Build history of the part. All positions in model axes, mm. A direction names the side the tool comes from. Give positions to 0.01 mm unless a question says otherwise; leave off trailing zeros. Loops run counter-clockwise (first coordinate to the right, second up) from the corner with the lowest first, then second, coordinate; pieces in that order, holes last. Notation, with made-up numbers: M 73,-22.75 L 100,-22.75 A14 ccw 100,-7.75 Z; hole C 30.5,-39 d4. An arc over 180 degrees is marked long. Answer as a JSON object with one key per item and string values. Group by question number.
1. Drill centre lines: line 1 along X through (y, z) = (16.5, -6.5); line 2 along Y through (x, z) = (62, -49); line 3 along Y through (x, z) = (69, -9). Where is each one in solid material? Low to high. Write a range as [from, to].
2. Mould opens along Z. For faces 4 (the face through (44, -4, -49.1)), 5 (the face through (44, -4, -20.9)), 6 (the face through (44, 7, 0)), 7 (the face through (90, 0.3, -6.4)) say: released by +Z, released by -Z, zero draft, split by the parting line, or undercut.
3. Slice it at A-A (y = 19.5). List the corners of the cut face in (x, z).
4. Drop flat-ended pins along their axis: pin 1 Ø4 at (x, z) = (78.5, -53) entering from -Y; pin 2 Ø21 at (x, z) = (59, -44) entering from +Y; pin 3 Ø2 at (x, z) = (68, -41.5) entering from -Y; pin 4 Ø14.5 at (y, z) = (16.5, -27.5) entering from +X. Give the stop position or say it passes through.
5. Slice it at B-B (z = -6). List the corners of the cut face in (x, y).
6. 3-axis set-ups, long thin cutter, end or side, ignore diameter. For faces 1 (the face through (90, 0.3, -42.2)), 2 (the face through (87, 2, -62.4)), 3 (the face through (44, -4, -72.1)): which of +Z, -Z, +X, -X, +Y, -Y reach the whole face in a straight line?
7. Slice it at C-C (y = -1). Give the number of separate pieces and of enclosed holes in the cut face, then the cut area to 3 significant figures.
from build123d import *

# Parameters (mm, degrees)
ESQUISSE1_W             = 90
ESQUISSE1_H             = 75
BOSS_EXTRU_1_DEPTH      = 3.7
ESQUISSE2_W             = 90
ESQUISSE2_H             = 2.9
ESQUISSE2_H_2           = 2
ESQUISSE2_H_3           = 0.8
BOSS_EXTRU_2_DEPTH      = 9
ENL_V_MAT_EXTRU_1_DEPTH = 118.84010353
ESQUISSE4_W             = 90
ESQUISSE4_H             = 2.9
BOSS_EXTRU_3_DEPTH      = 22
ESQUISSE5_W             = 72
ESQUISSE5_H             = 72.1
BOSS_EXTRU_4_DEPTH      = 20
CONG_1_R                = 1


with BuildPart() as part:
    # Esquisse1 → Boss.-Extru.1 (new body)
    with BuildSketch(Plane(origin=(0, 0, 0), x_dir=(1, 0, 0), z_dir=(0, 1, 0))):
        with Locations((45, 37.5)):
            Rectangle(ESQUISSE1_W, ESQUISSE1_H)
    extrude(amount=BOSS_EXTRU_1_DEPTH)

    # Esquisse2 → Boss.-Extru.2 (add)
    with BuildSketch(Plane.XZ):
        with Locations((45, -73.55)):
            Rectangle(ESQUISSE2_W, ESQUISSE2_H)
        with Locations((45, -1)):
            Rectangle(ESQUISSE2_W, ESQUISSE2_H_2)
        with Locations((45, -66.9)):
            Rectangle(ESQUISSE2_W, ESQUISSE2_H_3)
        with Locations((45, -61.1)):
            Rectangle(ESQUISSE2_W, ESQUISSE2_H_3)
        with Locations((45, -55.3)):
            Rectangle(ESQUISSE2_W, ESQUISSE2_H_3)
        with Locations((45, -49.5)):
            Rectangle(ESQUISSE2_W, ESQUISSE2_H_3)
        with Locations((45, -43.7)):
            Rectangle(ESQUISSE2_W, ESQUISSE2_H_3)
        with Locations((45, -37.9)):
            Rectangle(ESQUISSE2_W, ESQUISSE2_H_3)
        with Locations((45, -32.1)):
            Rectangle(ESQUISSE2_W, ESQUISSE2_H_3)
        with Locations((45, -26.3)):
            Rectangle(ESQUISSE2_W, ESQUISSE2_H_3)
        with Locations((45, -20.5)):
            Rectangle(ESQUISSE2_W, ESQUISSE2_H_3)
        with Locations((45, -14.7)):
            Rectangle(ESQUISSE2_W, ESQUISSE2_H_3)
        with Locations((45, -8.9)):
            Rectangle(ESQUISSE2_W, ESQUISSE2_H_3)
    extrude(amount=BOSS_EXTRU_2_DEPTH)

    # Esquisse3 → Enlèv. mat.-Extru.1 (cut, through all)
    with BuildSketch(Plane(origin=(0, 3.7, 0), x_dir=(1, 0, 0), z_dir=(0, 1, 0))):
        with BuildLine():
            Line((90, 12.6), (84.9, 12.6))
            ThreePointArc((84.9, 12.6), (82.5, 15), (84.9, 17.4))
            Line((84.9, 17.4), (90, 17.4))
            Line((90, 17.4), (90, 12.6))
        make_face()
        with BuildLine():
            Line((84.9, 57.6), (90, 57.6))
            Line((90, 57.6), (90, 62.4))
            Line((90, 62.4), (84.9, 62.4))
            ThreePointArc((84.9, 62.4), (82.5, 60), (84.9, 57.6))
        make_face()
        with BuildLine():
            Line((0, 57.6), (0, 62.4))
            Line((0, 62.4), (5.1, 62.4))
            ThreePointArc((5.1, 62.4), (7.5, 60), (5.1, 57.6))
            Line((5.1, 57.6), (0, 57.6))
        make_face()
        with BuildLine():
            Line((0, 17.4), (0, 12.6))
            Line((0, 12.6), (5.1, 12.6))
            ThreePointArc((5.1, 12.6), (7.5, 15), (5.1, 17.4))
            Line((5.1, 17.4), (0, 17.4))
        make_face()
    extrude(amount=-ENL_V_MAT_EXTRU_1_DEPTH, mode=Mode.SUBTRACT)

    # Esquisse4 → Boss.-Extru.3 (add)
    with BuildSketch(Plane(origin=(0, 3.7, 0), x_dir=(1, 0, 0), z_dir=(0, 1, 0))):
        with Locations((45, 73.55)):
            Rectangle(ESQUISSE4_W, ESQUISSE4_H)
    extrude(amount=BOSS_EXTRU_3_DEPTH)

    # Esquisse5 → Boss.-Extru.4 (add)
    with BuildSketch(Plane(origin=(0, 3.7, 0), x_dir=(1, 0, 0), z_dir=(0, 1, 0))):
        with Locations((45, 36.05)):
            Rectangle(ESQUISSE5_W, ESQUISSE5_H)
    extrude(amount=BOSS_EXTRU_4_DEPTH)

    # Congé1
    cong_1_edges = [part.edges().sort_by_distance(p)[0] for p in [
        (4.5, 3.7, 0),
        (85.5, 3.7, 0),
        (9, 3.7, -36.05),
        (81, 13.7, 0),
        (81, 3.7, -36.05),
        (81, 23.7, -36.05),
        (9, 13.7, 0),
        (45, 23.7, 0),
        (9, 23.7, -36.05),
    ]]
    fillet(cong_1_edges, radius=CONG_1_R)


solid = part.part
Established:
{
 "1": {"line 1": "x = [9, 81]", "line 2": "y = [0, 23.7]", "line 3": "y = [-9, 23.7]"},
 "2": {"face 4": "undercut", "face 5": "undercut", "face 6": "released by +Z", "face 7": "zero draft"},
 "3": {"outline": "M 0,-75 L 90,-75 L 90,-72.1 L 81,-72.1 L 81,-1 A1 ccw 80,0 L 10,0 A1 ccw 9,-1 L 9,-72.1 L 0,-72.1 Z"},
 "4": {"pin 1": "stops at y = -9", "pin 2": "stops at y = 23.7", "pin 3": "stops at y = 0", "pin 4": "stops at x = 81"},
 "5": {"outline": "M 0,0 L 90,0 L 90,3.7 L 82,3.7 A1 cw 81,4.7 L 81,22.7 A1 ccw 80,23.7 L 10,23.7 A1 ccw 9,22.7 L 9,4.7 A1 cw 8,3.7 L 0,3.7 Z"},
 "6": {"face 1": "+Z, -Z, +X, +Y, -Y", "face 2": "+X, +Y, -Y", "face 3": "+X, -X, -Y"},
 "7": {"separate pieces": "13", "enclosed holes": "0", "area": "1,210 mm^2"}
}
